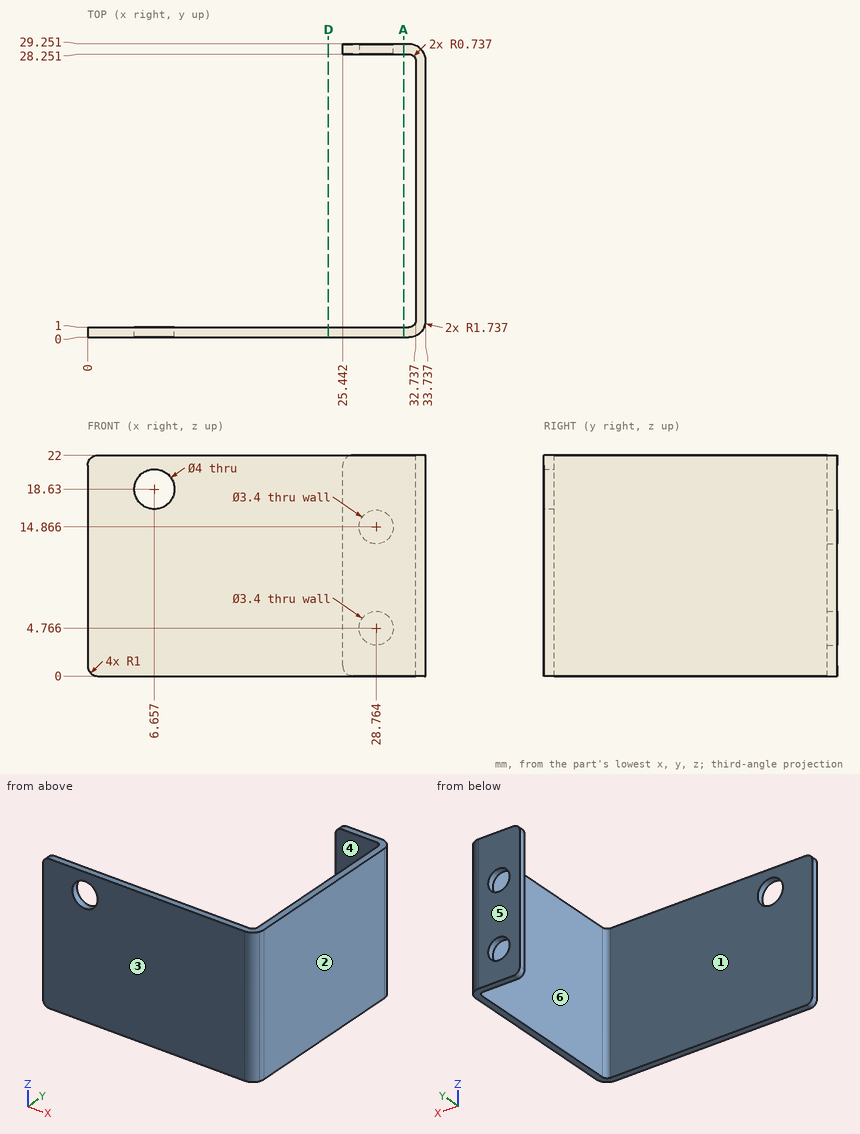
For this review, use the dimensioned drawing (mm, ordinates from the lowest corner) and the shaded views. A direction names the side the tool comes from. Round coordinates to 2 decimals unless told otherwise and drop trailing zeros. Write each loop counter-clockwise with the first axis right and the second up, starting at its lowest first coordinate (ties: lowest second). Pieces come first, ordered by that corner, then holes. Notation, with made-up numbers: (-33.5, 3) -> (6.5, 3) arc R23 cw to (6.5, 41) -> close; hole circle Ø6 at (89.5, 61.5). An arc over 180 degrees is marked (long way). Use CSV: the item, a comma, the result in double quotes.
Q1. For the marked faces 1 and 2, list the 3-axis set-ups (+Z, -Z, +X, -X, +Y, -Y) from which the entire face can be reached by the end or side of a thin tool; tool diameter is ignored.
Checks:
face 1,"+Z, -Z, -X"
face 2,"+Z, -Z, +X, +Y, -Y"
Q2. For pin 1 Ø4 at (y, z) = (22, 10) entering from -X; pin 2 Ø2 at (x, z) = (28.76, 14.87) entering from +Y; pin 3 Ø0.8 at (y, z) = (28.5, 8) entering from -X, all flat-tipped, find the tip position at first contact; note any pin that passes through.
Checks:
pin 1,"x = 32.74"
pin 2,"y = 1"
pin 3,"x = 25.44"
Q3. To check wall thickness, follow probe 1 along Y at (x, z) = (31, 20); probe 2 along Y at (x, z) = (25, 21.25); probe 3 along X at (y, z) = (15.5, 18.5). State the ranges of each line that lie inside material, in increasing order. Write a range as [from, to].
Checks:
probe 1,"[0, 1], [28.25, 29.25]"
probe 2,"[0, 1]"
probe 3,"[32.74, 33.74]"
Q4. Consider section D-D (x = 24). Give the boundary of the cut face in (y, z).
Checks:
outline,"(0, 0) -> (1, 0) -> (1, 22) -> (0, 22) -> close"
Q5. Consider section A-A (x = 31.5). Give the boundary of the cut face in (y, z).
Checks:
outline,"(0, 0) -> (1, 0) -> (1, 22) -> (0, 22) -> close; (28.25, 0) -> (29.25, 0) -> (29.25, 22) -> (28.25, 22) -> close"
Q6. Mouldability with a two-part tool opening along Y and no side actions: class the marked faces 3, 4, 5 and 6 as released by +Y, released by -Y, zero draft, split by the parting line, or undercut.
Checks:
face 3,"released by -Y"
face 4,"undercut"
face 5,"released by +Y"
face 6,"undercut"
